```python
from build123d import *

# Parameters (mm, degrees)
F1_DEPTH        = 20
F2_R            = 10
F3_R            = 10
F4_R            = 5
F5_R            = 5
F6_R            = 5
F7_R            = 5
F8_R            = 1
F10_D           = 4
F10_CSINK_D     = 7
F10_CSINK_ANGLE = 90


with BuildPart() as f1:
    # F0 (on Front) → F1 (new body)
    with BuildSketch(Plane.XZ):
        Polygon((33.675430585, 61.2683971646), (-35.6066017178, 21.2683971646), (-35.6066017178, -33.7316028354), (-35.6066017178, -38.7316028354), (-30.6066017178, -38.7316028354), (-10.6066017178, -38.7316028354), (0, -28.1250011176), (-3.5355339059, -24.5894672117), (-12.6776695297, -33.7316028354), (-30.6066017178, -33.7316028354), (-30.6066017178, 18.3816458187), (36.175430585, 56.9382701457), align=None)
    extrude(amount=F1_DEPTH)

    # F2
    f2_edges = [f1.edges().sort_by_distance(p)[0] for p in [
        (-35.606602, -10, 21.268397),
    ]]
    fillet(f2_edges, radius=F2_R)

    # F3
    f3_edges = [f1.edges().sort_by_distance(p)[0] for p in [
        (-35.606602, -10, -38.731603),
        (-10.606602, -10, -38.731603),
    ]]
    fillet(f3_edges, radius=F3_R)

    # F4
    f4_edges = [f1.edges().sort_by_distance(p)[0] for p in [
        (-30.606602, -10, -33.731603),
        (-12.67767, -10, -33.731603),
    ]]
    fillet(f4_edges, radius=F4_R)

    # F5
    f5_edges = [f1.edges().sort_by_distance(p)[0] for p in [
        (-30.606602, -10, 18.381646),
    ]]
    fillet(f5_edges, radius=F5_R)

    # F6
    f6_edges = [f1.edges().sort_by_distance(p)[0] for p in [
        (-1.767767, 0, -26.357234),
        (-1.767767, -20, -26.357234),
    ]]
    fillet(f6_edges, radius=F6_R)

    # F7
    f7_edges = [f1.edges().sort_by_distance(p)[0] for p in [
        (34.925431, 0, 59.103334),
        (34.925431, -20, 59.103334),
    ]]
    fillet(f7_edges, radius=F7_R)

    # F8
    f8_edges = [f1.edges().sort_by_distance(p)[0] for p in [
        (-0.630649, -20, 41.461773),
        (1.869351, -20, 37.131646),
        (32.407166, -18.535534, 60.536164),
        (34.907166, -18.535534, 56.206037),
    ]]
    fillet(f8_edges, radius=F8_R)

    # F10 (through all)
    with Locations(Plane.YZ.offset(-30.6066017178)):
        with Locations((-13, 5.4948944727), (-7, -8.7316028354)):
            CounterSinkHole(F10_D / 2, F10_CSINK_D / 2, counter_sink_angle=F10_CSINK_ANGLE)


solid = f1.part
```
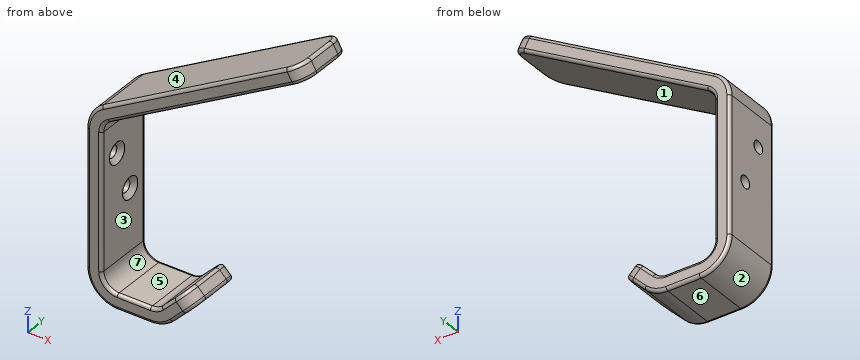
Part model, mm, in its own coordinate system. Face numbers are marked on the shaded views. A direction names the side the tool comes from. Round coordinates to 2 decimals unless told otherwise and drop trailing zeros. Write each loop counter-clockwise with the first axis right and the second up, starting at its lowest first coordinate (ties: lowest second). Pieces come first, ordered by that corner, then holes. Notation, with made-up numbers: M -35.5,40 L 17.5,40 A7 cw 17.5,53 Z; hole C 88,43 d11. An arc over 180 degrees is marked long. Answer as CSV lines item,"result". Start each with the question number.
1) Which spindle directions (+Z, -Z, +X, -X, +Y, -Y) get a long thin tool onto all of the face, cutting with end or side? Do the marked faces 1, 2 and 3. Say none if no direction does.
2) Band-saw the part on B-B (z = -19). List the corners of the cut face in (x, y), then the cut area to 3 significant figures.
3) Drill centre lines: L1, parallel to X at y = -7.5, z = -20; L2, parallel to Z at x = -7.5, y = -13 (3 decimals); L3, parallel to Z at x = -15, y = -13. Where is each one in solid material? Low to high.
4) Mould opens along X. For the marked faces 4, 5, 6 and 7 say: +X half, -X half, draft (parallel to the pull), parting line (faces both ways), or undercut.
5) Drop flat-ended pins along their axis: pin 1 (5 mm diameter, centred on y = -12.5, z = 33, fed in from +X); pin 2 (5.5 mm diameter, centred on x = -19, y = -9.5, fed in from +Z); pin 3 (5 mm diameter, centred on x = 12, y = -7.5, fed in from +Z); pin 4 (3 mm diameter, centred on y = -7, z = -8.73, fed in from +X). Give the stop position or say it passes through.
6) Band-saw the part on A-A (y = -13). List the corners of the cut face in (x, z) (3 decimals), then the cut area to 3 significant figures.
Worked out:
1,face 1,"+X, +Y, -Y"
1,face 2,"-Z, -X, +Y, -Y"
1,face 3,"+Y, -Y"
2,outline,"M -35.61,-19 A1 ccw -34.61,-20 L -31.61,-20 A1 ccw -30.61,-19 L -30.61,-1 A1 ccw -31.61,0 L -34.61,0 A1 ccw -35.61,-1 Z"
2,area,"99.1 mm²"
3,L1,"-35.61 to -30.61"
3,L2,"-35.625 to -28.554, 31.722 to 37.496"
3,L3,"-38.73 to -33.73, 27.39 to 33.17"
4,face 4,"-X half"
4,face 5,"undercut"
4,face 6,"draft"
4,face 7,"undercut"
5,pin 1,"x = -0.96"
5,pin 2,"z = 32.44"
5,pin 3,"z = 50.2"
5,pin 4,"through"
6,outline,"M -35.607,-28.732 A10 ccw -25.607,-38.732 L -14.749,-38.732 A10 ccw -7.678,-35.803 L -0.707,-28.832 A1 ccw -0.707,-27.418 L -2.828,-25.297 A1 ccw -4.243,-25.297 L -11.213,-32.267 A5 cw -14.749,-33.732 L -25.607,-33.732 A5 cw -30.607,-28.732 L -30.607,1.995 L -32.107,3.495 L -35.607,3.495 Z; M -35.607,7.495 L -32.107,7.495 L -30.607,8.995 L -30.607,15.495 A5 cw -28.107,19.825 L 35.309,56.438 A1 ccw 35.675,57.804 L 34.175,60.402 A1 ccw 32.809,60.768 L -30.607,24.155 A10 ccw -35.607,15.495 Z"
6,area,"805 mm²"
